Autodesk Inventor part; units mm, degrees
ref_plane "YZ Plane" through (0, 0, 0) normal (1, 0, 0) x (0, 1, 0)
ref_plane "XZ Plane" through (0, 0, 0) normal (0, 1, 0) x (-1, 0, 0)
ref_plane "XY Plane" through (0, 0, 0) normal (0, 0, 1) x (1, 0, 0)
sketch "Sketch1" plane through (0, 0, 0) normal (0, 1, 0) x (-1, 0, 0)
  arc A0 (0, -3.4) -> (0, 3.4) centre (0, 0) ccw
  line L0 (0, 3.4) -> (-10, 3.4)
  line L1 (-10, 3.4) -> (-10, -3.4)
  line L2 (-10, -3.4) -> (0, -3.4)
  line L3 (0, 3.4) -> (0, -3.4)
  dimension "d0" = 10
  dimension "d1" = 6.8
extrude "Extrusion1" add sketch "Sketch1" along normal blind 9
sketch "Sketch2" plane through (0, 9, 0) normal (0, 1, 0) x (1, 0, 0)
  line L0 (9, -3.4) -> (10, -3.4)
  arc A0 (9, -3.4) -> (10, -3.4) centre (9.5, -3.4) ccw
  point P0 (0, 0)
  dimension "d4" = 1
extrude "Extrusion2" add sketch "Sketch2" against normal blind 9
pattern_linear "Rectangular Pattern1" count 5 spacing 2 along (-1, 0, 0) of "Extrusion2"
sketch "Sketch3" plane through (10, 0, -3.4) normal (1, 0, 0) x (0, 0, -1)
  line L0 (-3.4, 0) -> (-3.4, 9)
  line L1 (0, 9) -> (-6.8, 9)
  circle A0 centre (-3.4, 4.5) radius 1.7
  dimension "d10" = 3.4
extrude "Extrusion3" cut sketch "Sketch3" against normal blind 4
properties part number "XY_Tensioner" material "ABS Plastic"
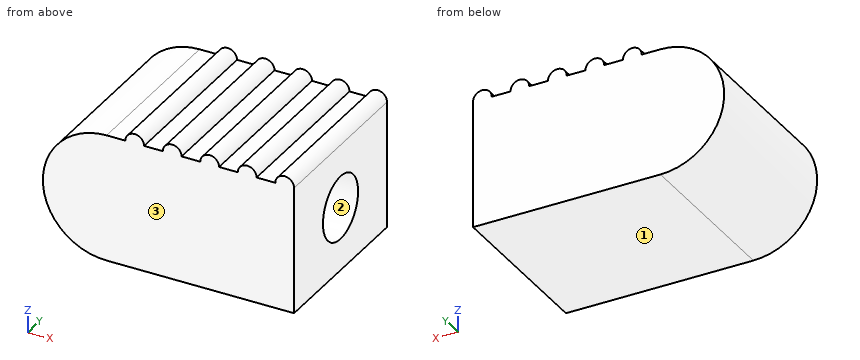
The listing builds one solid part. Answer for the finished solid, in the listing's coordinates (mm). Face numbers are marked on the shaded views. Give positions to 0.01 mm unless a question says otherwise; leave off trailing zeros. Order: outer loops, then holes, each group sorted by start corner. A loop starts at its lowest first (then second) coordinate and runs counter-clockwise, first axis right, second up. Notation, with made-up numbers: (80, -35.5) -> (108, -35.5) arc R20 cw to (108, 3.5) -> close; hole circle Ø10 at (11.5, -26). An arc over 180 degrees is marked (long way). Answer as CSV lines item,"result". Start each with the question number.
Q1. Determine the mould class of the marked faces 1, 2 and 3 for opening direction Y: pulls with the +Y half, pulls with the -Y half, needs draft (parallel to the pull), parting line crosses it, or undercut.
Q2. Find the intervals of material crossed by L1, parallel to Z at x = 8.25, y = 4.5; L2, parallel to Y at x = 7.65, z = 0; L3, parallel to Z at x = 7.55, y = 4.5, in increasing order.
Q3. Given pin 1 (1 mm diameter, centred on y = 3.5, z = 3, fed in from -X); pin 2 (0.8 mm diameter, centred on x = 2.5, y = 3, fed in from +Z), each flat-ended and moving along its own axis, determine where each tip first touches the part or whether it passes through.
Q4. A cutting plane is placed at C-C (y = 0.5). Determine the outline of the cut face in (x, z), then the cut area to 3 significant figures.
Q5. A cutting plane is placed at D-D (x = 2.5). Determine the outline of the cut face in (y, z).
Q6. A cutting plane is placed at A-A (z = 0). Determine the outline of the cut face in (x, y), then the cut area to 3 significant figures.
Q7. A cutting plane is placed at B-B (x = 7.5). Determine the outline of the cut face in (y, z).
Results found:
1,face 1,"needs draft"
1,face 2,"undercut"
1,face 3,"pulls with the -Y half"
2,L1,"-3.4 to -1.7, 1.7 to 3.4"
2,L2,"0 to 2.8, 6.2 to 9"
2,L3,"-3.4 to -1.7, 1.7 to 3.9"
3,pin 1,"x = -2.3"
3,pin 2,"z = 3.4"
4,outline,"(0, -3.4) -> (10, -3.4) -> (10, 3.4) arc R0.5 ccw to (9, 3.4) -> (8, 3.4) arc R0.5 ccw to (7, 3.4) -> (6, 3.4) arc R0.5 ccw to (5, 3.4) -> (4, 3.4) arc R0.5 ccw to (3, 3.4) -> (2, 3.4) arc R0.5 ccw to (1, 3.4) -> (0, 3.4) arc R3.4 ccw to start"
4,area,"88.1 mm2"
5,outline,"(0, -3.4) -> (9, -3.4) -> (9, 3.4) -> (0, 3.4) -> close"
6,outline,"(-3.4, 0) -> (10, 0) -> (10, 2.8) -> (6, 2.8) -> (6, 6.2) -> (10, 6.2) -> (10, 9) -> (-3.4, 9) -> close"
6,area,"107 mm2"
7,outline,"(0, -3.4) -> (9, -3.4) -> (9, 3.9) -> (0, 3.9) -> close; hole circle Ø3.4 at (4.5, 0)"
